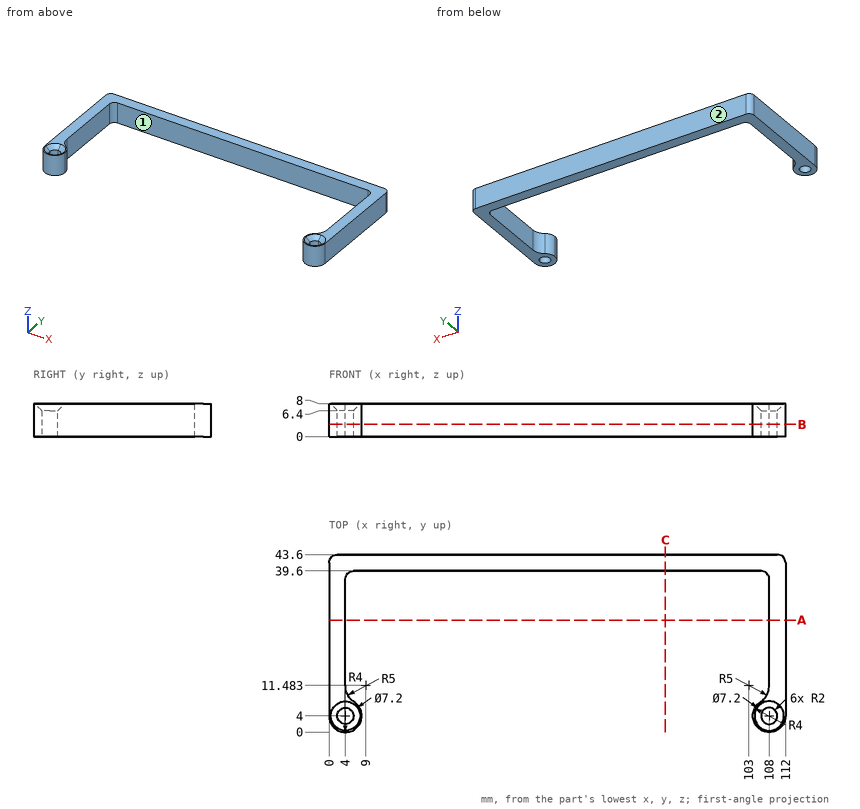
Geometry: see drawing. Coordinates: mm, zero at the bounding-box minimum. Coordinates: 2 decimals unless noted, no trailing zeros. Loops run counter-clockwise (first coordinate to the right, second up) from the corner with the lowest first, then second, coordinate; pieces in that order, holes last.
Q1. Contact query for a flat-ended pin moving along its axis: pin 1 (4 mm diameter, centred on x = 55.5, z = 4.5, fed in from -Y). Output: stop coordinate, or through.
Q2. Material intervals for line 1 (X direction, y = 33.5, z = 1.5); line 2 (X direction, y = 5.5, z = 7) (1 decimal); line 3 (Y direction, x = 107, z = 2) (1 decimal), sorted ascending.
Q3. Cut plane C-C (x = 82.5). Output: boundary loops of the cut face in (y, z).
Q4. Draft query along X for the marked faces 1 and 2. Return one class per face: +X half, -X half, draft (parallel to the pull), parting line (faces both ways), or undercut.
Q5. Cut plane B-B (z = 3). Output: boundary loops of the cut face in (x, y).
Q6. Cut plane A-A (y = 27.5). Output: boundary loops of the cut face in (x, z).
Working result:
1. pin 1: stops at y = 39.6
2. line 1: x = 0 to 4, 108 to 112
2. line 2: x = 0 to 1.9, 6.1 to 7.7, 104.3 to 105.9, 110.1 to 112
2. line 3: y = 0.1 to 2.3, 5.7 to 8.5, 39.3 to 43.6
3. outline: (39.6, 0) - (43.6, 0) - (43.6, 8) - (39.6, 8) - close
4. face 1: undercut
4. face 2: draft
5. outline: (0, 4) arc R4 ccw (long way) to (6.22, 7.33) arc R5 cw to (4, 11.48) - (4, 37.6) arc R2 cw to (6, 39.6) - (106, 39.6) arc R2 cw to (108, 37.6) - (108, 11.48) arc R5 cw to (105.78, 7.33) arc R4 ccw (long way) to (112, 4) - (112, 41.6) arc R2 ccw to (110, 43.6) - (2, 43.6) arc R2 ccw to (0, 41.6) - close; hole circle Ø4 at (4, 4); hole circle Ø4 at (108, 4)
6. outline: (0, 0) - (4, 0) - (4, 8) - (0, 8) - close; (108, 0) - (112, 0) - (112, 8) - (108, 8) - close
